Autodesk Inventor part; units mm, degrees
ref_plane "YZ Plane" through (0, 0, 0) normal (1, 0, 0) x (0, 1, 0)
ref_plane "XZ Plane" through (0, 0, 0) normal (0, 1, 0) x (-1, 0, 0)
ref_plane "XY Plane" through (0, 0, 0) normal (0, 0, 1) x (1, 0, 0)
sketch "草图1" plane through (0, 0, 0) normal (0, 1, 0) x (-1, 0, 0)
  line L0 (34.5, 19.3) -> (-34.5, 19.3)
  line L1 (-34.5, 19.3) -> (-34.5, -19.3)
  line L2 (-34.5, -19.3) -> (34.5, -19.3)
  line L3 (34.5, -19.3) -> (34.5, 19.3)
  circle A0 centre (29.7, 14.5) radius 4.8
  line L4 (48.3, 0) -> (-48.3, 0)
  line L5 (0, -27.02) -> (0, 27.02)
  circle A1 centre (29.7, -14.5) radius 4.8
  circle A2 centre (-29.7, 14.5) radius 4.8
  circle A3 centre (-29.7, -14.5) radius 4.8
  point P0 (0, 0)
  dimension "d0" = 38.6
  dimension "d1" = 69
  dimension "d2" = 34.5
  dimension "d3" = 19.3
  dimension "d4" = 9.6
extrude "拉伸1" add sketch "草图1" along normal blind 4
extrude "拉伸2" add sketch "草图1" against normal blind 8 contours A0 | A2 | A1 | A3
sketch "草图2" plane through (0, 0, 0) normal (0, 0, 1) x (1, 0, 0)
  line L0 (24.9, -8) -> (34.5, -8)
  line L1 (34.5, 0) -> (29.7, 0)
  line L2 (29.7, 0) -> (34.5, 0)
  line L3 (34.5, 0) -> (34.5, -8)
  line L4 (34.5, -4.8) -> (32, -4.8)
  line L5 (32, -4.8) -> (32, -1.8)
  line L6 (32, -1.8) -> (34.5, -1.8)
  line L7 (34.5, -1.8) -> (34.5, -4.8)
  point P0 (0, 0)
  dimension "d9" = 1.8
  dimension "d10" = 3
  dimension "d11" = 2.5
extrude "拉伸3" [suppressed]
mirror "镜像1" [suppressed]
sketch "草图3" plane through (29.7, -8, -14.5) normal (0, -1, 0) x (1, 0, 0)
  arc A0 (2.3, -4.2131) -> (2.3, 4.2131) centre (0, 0) ccw
  circle A1 centre (0, 0) radius 4.8
  line L0 (0, 0) -> (0, -4.8)
  line L1 (-2.5, -1.8) -> (2.5, -1.8)
  line L2 (2.5, -1.8) -> (2.5, -4.8)
  line L3 (2.5, -4.8) -> (-2.5, -4.8)
  line L4 (-2.5, -4.8) -> (-2.5, -1.8)
  line L5 (4.8, -4.8) -> (0, -4.8)
  point P0 (-29.7, 14.5)
  point P1 (2.4, -4.8)
  dimension "d17" = 2.5
  dimension "d18" = 5
  dimension "d19" = 3
extrude "拉伸4" cut sketch "草图3" against normal through all contours L2 L3 A1 A0 | A0 A1 L0 L1 L2 | L4 L1 L0 A1 | A1 L3 L4
sketch "草图4" plane through (0, 4, 0) normal (0, 1, 0) x (1, 0, 0)
  line L0 (-48.3, 0) -> (48.3, 0)
  line L1 (0, 27.02) -> (0, -27.02)
  line L2 (28.3221, -16.1643) -> (19.8368, -7.679)
  line L3 (19.8368, -7.679) -> (23.3723, -4.1435)
  line L4 (23.3723, -4.1435) -> (31.8576, -12.6288)
  line L5 (31.8576, -12.6288) -> (28.3221, -16.1643)
  line L6 (34.5, -19.3) -> (17.3206, -2.1206)
  line L7 (-28.3221, -16.1643) -> (-19.8368, -7.679)
  line L8 (-19.8368, -7.679) -> (-23.3723, -4.1435)
  line L9 (-23.3723, -4.1435) -> (-31.8576, -12.6288)
  line L10 (-31.8576, -12.6288) -> (-28.3221, -16.1643)
  line L11 (28.3221, 16.1643) -> (19.8368, 7.679)
  line L12 (19.8368, 7.679) -> (23.3723, 4.1435)
  line L13 (23.3723, 4.1435) -> (31.8576, 12.6288)
  line L14 (31.8576, 12.6288) -> (28.3221, 16.1643)
  line L15 (-28.3221, 16.1643) -> (-19.8368, 7.679)
  line L16 (-23.3723, 4.1435) -> (-31.8576, 12.6288)
  line L17 (-31.8576, 12.6288) -> (-28.3221, 16.1643)
  line L18 (-19.8368, 7.679) -> (-23.3723, 4.1435)
  point P0 (0, 0)
  dimension "d22" = 5
  dimension "d23" = 12
extrude "拉伸5" add sketch "草图4" along normal blind 10
sketch "草图5" plane through (19.8368, 4, -7.679) normal (-0.7071, 0, -0.7071) x (-0.7071, 0, 0.7071)
  line L0 (0, 0) -> (-12, 0)
  line L1 (0, 0) -> (0, 10)
  line L2 (-12, 10) -> (0, 10)
  line L3 (-12, 0) -> (-12, 10)
  circle A0 centre (-6, 5) radius 1.5
  line L4 (-12, 10) -> (0, 10)
  line L5 (-6, 10) -> (-6, 0)
  point P0 (19.4566, -4)
  dimension "d26" = 3
  dimension "d27" = 5
extrude "拉伸6" cut sketch "草图5" against normal blind 10 contours L5 A0 | A0 L5
mirror "镜像2" about plane through (0, 0, 0) normal (1, 0, 0) of "拉伸6"
mirror "镜像3" about plane through (0, 0, 0) normal (0, 0, 1) of "拉伸6"
mirror "镜像4" about plane through (0, 0, 0) normal (1, 0, 0) of "拉伸6", "镜像3"
sketch "草图6" plane through (0, 0, 0) normal (1, 0, 0) x (0, 1, 0)
  line L0 (-4.8, 16.8) -> (-1.8, 16.8)
  line L1 (-1.8, 16.8) -> (-1.8, 19.3)
  line L2 (-1.8, 19.3) -> (-4.8, 19.3)
  line L3 (-4.8, 19.3) -> (-4.8, 16.8)
  line L4 (0, 19.3) -> (-8.1735, 19.3)
  line L5 (0, 19.3) -> (0, 15.2583)
  point P0 (0, 0)
  point P1 (-3.3, 19.3)
  dimension "d30" = 3
  dimension "d31" = 2.5
  dimension "d32" = 1.8
extrude "拉伸7" cut sketch "草图6" along normal through all both and the other way through all
mirror "镜像5" about plane through (0, 0, 0) normal (0, 0, 1) of "拉伸7"
properties part number "landframe"
Can you work these out from the model? Positions are in its coordinate system, mm. A direction names the side the tool comes from. Round coordinates to 2 decimals unless told otherwise and drop trailing zeros. Loops run counter-clockwise (first coordinate to the right, second up) from the corner with the lowest first, then second, coordinate; pieces in that order, holes last. Notation, with made-up numbers: M -36,-40 L 0,-40 A36 ccw 0,-4 Z; hole C 9.5,80 d3. An arc over 180 degrees is marked long. Answer as a JSON object with one key per item and string values. Group by question number.
Q1. Will these pins go through, and if not, where does the flat tip stop? pin 1 (0.9 mm diameter, centred on x = 26.5, z = -17.5, fed in from +Y); pin 2 (1.9 mm diameter, centred on x = 26.5, y = -3.5, fed in from -Z); pin 3 (5 mm diameter, centred on x = -27.5, z = -7, fed in from +Y); pin 4 (4 mm diameter, centred on x = 29, y = -1.5, fed in from -Z).
Q2. Please list where these lines run through material, in increasing order: L1, parallel to Y at x = 14, z = 3.5; L2, parallel to Y at x = -30, z = -10; L3, parallel to Z at x = -24, y = 5.5.
Q3. On a 3-axis mill with a long thin cutter (end or side, diameter ignored), from which of +Z, -Z, +X, -X, +Y, -Y can I reach the whole of each face in a straight line? I mean faces 1 (the flat face through (-28.5, 7.82, 9.27)), 2 (the flat face through (28.5, 7.82, -9.27)), 3 (the flat face through (34, 0, -18)), 4 (the flat face through (-25.08, 10.04, -12.92)). Say none if no direction works.
Q4. Imagine slicing it at B-B, the plane x = 6.5. Please give me the cut outline in (y, z).
Q5. Imagine slicing it at C-C, the plane z = 15.5. Please give me the cut outline in (x, y).
Q6. Imagine slicing it at A-A, the plane y = 11.75. Please give me the cut outline in (x, z), then the cut area to 3 significant figures.
Q7. We'd pull the mould along Z, two halves only. Please class faces 5 (the flat face through (-34.5, 2, 0)), 6 (the flat face through (0, 4, 0)), 7 (the flat face through (30.115, 8.93, 14.372)): +Z half, -Z half, draft (parallel to the pull), parting line (faces both ways), or undercut.
Findings:
{
 "1": {"pin 1": "stops at y = 4", "pin 2": "stops at z = -16.8", "pin 3": "stops at y = 14", "pin 4": "stops at z = -18.6"},
 "2": {"L1": "y = 0 to 4", "L2": "y = -8 to 4", "L3": "z = -11.84 to -4.77, 4.77 to 11.84"},
 "3": {"face 1": "-X, +Y", "face 2": "+X, +Y", "face 3": "-Z, +X, -Y", "face 4": "-Z, +Y"},
 "4": {"outline": "M 0,-19.3 L 4,-19.3 L 4,19.3 L 0,19.3 Z"},
 "5": {"outline": "M -34.5,0 L -34.39,0 L -34.39,-8 L -25.01,-8 L -25.01,0 L 25.01,0 L 25.01,-8 L 34.39,-8 L 34.39,0 L 34.5,0 L 34.5,4 L 28.99,4 L 28.99,14 L 27.66,14 L 27.66,4 L -27.66,4 L -27.66,14 L -28.99,14 L -28.99,4 L -34.5,4 Z"},
 "6": {"outline": "M -31.86,-12.63 L -28.32,-16.16 L -19.84,-7.68 L -23.37,-4.14 Z; M -31.86,12.63 L -23.37,4.14 L -19.84,7.68 L -28.32,16.16 Z; M 19.84,-7.68 L 28.32,-16.16 L 31.86,-12.63 L 23.37,-4.14 Z; M 19.84,7.68 L 23.37,4.14 L 31.86,12.63 L 28.32,16.16 Z", "area": "240 mm2"},
 "7": {"face 5": "draft", "face 6": "undercut", "face 7": "+Z half"}
}
